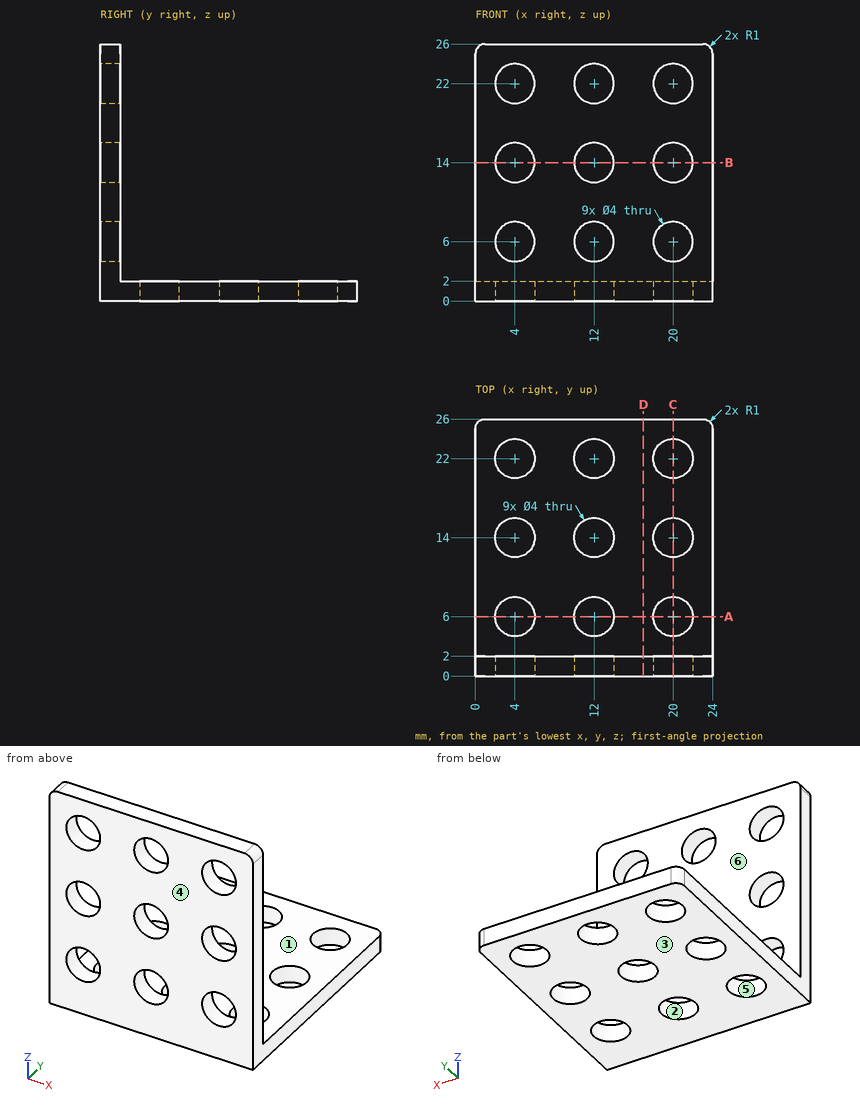
Here's the drawing with two shaded views (mm, measured from the low corner). I have some questions. A direction names the side the tool comes from. Give positions to 0.01 mm unless a question says otherwise; leave off trailing zeros. Loops run counter-clockwise (first coordinate to the right, second up) from the corner with the lowest first, then second, coordinate; pieces in that order, holes last. Notation, with made-up numbers: (85, 42.25) -> (114, 42.25) arc R13 cw to (114, 58.25) -> close; hole circle Ø1 at (-7, 9). An arc over 180 degrees is marked (long way). Answer as a JSON object with one key per item and string values. Group by question number.
Item 1: Imagine slicing it at A-A on y = 6. Write out the boundary of the cut face in (x, z).
Item 2: I need wall thicknesses on L1, parallel to X at y = 6, z = 1.4; L2, parallel to Z at x = 11.25, y = 1.5; L3, parallel to Y at x = 10.25, z = 9.25. Which ranges of each line are inside material? Lowest first, please.
Item 3: On a 3-axis mill with a long thin cutter (end or side, diameter ignored), from which of +Z, -Z, +X, -X, +Y, -Y can I reach the whole of each face in a straight line? I mean the marked faces 1 and 2. Say none if no direction works.
Item 4: Will these pins go through, and if not, where does the flat tip stop? pin 1 (5 mm diameter, centred on x = 4, y = 22, fed in from -Z); pin 2 (6.5 mm diameter, centred on x = 4, y = 14, fed in from +Z); pin 3 (6.5 mm diameter, centred on x = 20, z = 22, fed in from +Y).
Item 5: Thinking about a two-plate mould opening in Y: for the marked faces 3, 4, 5 and 6, which applies, pulls with the +Y half, pulls with the -Y half, needs draft (parallel to the pull), parting line crosses it, or undercut?
Item 6: Imagine slicing it at C-C on x = 20. Give the number of separate pieces and of enclosed holes in the cut face, then the cut area to 3 significant figures.
Item 7: Imagine slicing it at D-D on x = 17. Write out the boundary of the cut face in (y, z), then the cut area to 3 significant figures.
Answer list:
{
 "1": {"outline": "(0, 0) -> (2, 0) -> (2, 2) -> (0, 2) -> close; (6, 0) -> (10, 0) -> (10, 2) -> (6, 2) -> close; (14, 0) -> (18, 0) -> (18, 2) -> (14, 2) -> close; (22, 0) -> (24, 0) -> (24, 2) -> (22, 2) -> close"},
 "2": {"L1": "x = 0 to 2, 6 to 10, 14 to 18, 22 to 24", "L2": "z = 0 to 4.15, 7.85 to 12.15, 15.85 to 20.15, 23.85 to 26", "L3": "y = 0 to 2"},
 "3": {"face 1": "+Z, +X, -X, +Y", "face 2": "+Z, -Z"},
 "4": {"pin 1": "stops at z = 0", "pin 2": "stops at z = 2", "pin 3": "stops at y = 2"},
 "5": {"face 3": "needs draft", "face 4": "pulls with the -Y half", "face 5": "undercut", "face 6": "pulls with the +Y half"},
 "6": {"separate pieces": "7", "enclosed holes": "0", "area": "52.0 mm2"},
 "7": {"outline": "(0, 0) -> (26, 0) -> (26, 2) -> (2, 2) -> (2, 26) -> (0, 26) -> close", "area": "100 mm2"}
}
